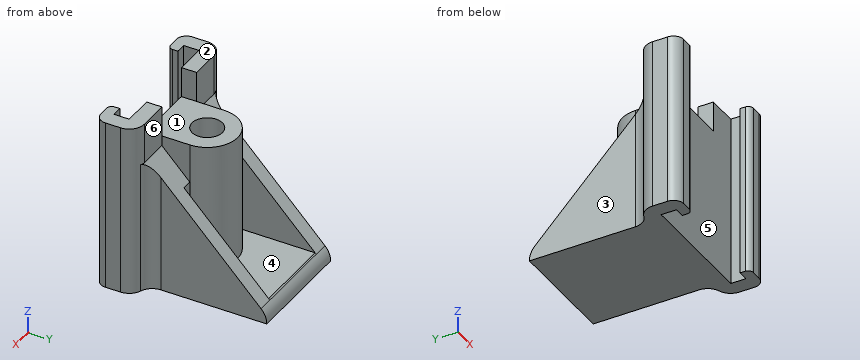
from build123d import *

# Parameters (mm, degrees)
BOSS_EXTRUDE1_DEPTH   = 107.95
BOSS_EXTRUDE1_2_DEPTH = 107.95
SKETCH1_6_W           = 6.35
SKETCH1_6_H           = 17.4625
BOSS_EXTRUDE2_DEPTH   = 82.55
CUT_EXTRUDE2_REACH    = 157.031
BOSS_EXTRUDE4_DEPTH   = 88.9
BOSS_EXTRUDE6_REACH   = 152.176
SKETCH5_R             = 9.525
CUT_EXTRUDE3_DEPTH    = 31.75
FILLET2_R             = 9.525


with BuildPart() as part:
    # Sketch1 → Boss-Extrude1 (new body)
    with BuildSketch(Plane.XY):
        with BuildLine():
            ThreePointArc((34.925, -25.4), (32.67993597, -24.47006403), (31.75, -22.225))
            Line((31.75, -22.225), (31.75, -19.05))
            Line((31.75, -19.05), (38.1, -19.05))
            Line((38.1, -19.05), (38.1, -9.525))
            Line((38.1, -9.525), (19.05, -9.525))
            Line((19.05, -9.525), (19.05, 0))
            Line((19.05, 0), (38.1, 0))
            ThreePointArc((38.1, 0), (44.835192091, -2.789807909), (47.625, -9.525))
            Line((47.625, -9.525), (47.625, -19.05))
            ThreePointArc((47.625, -19.05), (45.765128061, -23.540128061), (41.275, -25.4))
            Line((41.275, -25.4), (34.925, -25.4))
        make_face()
    extrude(amount=BOSS_EXTRUDE1_DEPTH)

    # Sketch1<6> → Boss-Extrude2 (add)
    with BuildSketch(Plane.XY):
        with Locations((22.225, 8.73125)):
            Rectangle(SKETCH1_6_W, SKETCH1_6_H)
        Polygon((25.4, 17.4625), (25.4, 0), (34.925, 0), (34.925, 74.6125), (25.4, 74.6125), align=None)
    boss_extrude2 = extrude(amount=BOSS_EXTRUDE2_DEPTH)

    # Cut-Extrude2: up to this face of the body (flat: up to its plane)
    cut_extrude2_end = Plane(part.part.faces().sort_by_distance((19.05, 3.113443878, 46.562346939))[0])
    # Sketch3 → Cut-Extrude2 (cut, up to the picked face)
    with BuildSketch(Plane(origin=(34.925, 0, 0), x_dir=(0, 0, -1), z_dir=(1, 0, 0)), mode=Mode.PRIVATE) as cut_extrude2_sk1:
        with BuildLine():
            Line((-82.55, 0), (-8.812527697, 71.057408725))
            ThreePointArc((-8.812527697, 71.057408725), (-4.751297675, 73.690240462), (0, 74.6125))
            Line((0, 74.6125), (-82.55, 74.6125))
            Line((-82.55, 74.6125), (-82.55, 0))
        make_face()
    cut_extrude2_tool1 = split(extrude(cut_extrude2_sk1.sketch, amount=-CUT_EXTRUDE2_REACH, mode=Mode.PRIVATE), bisect_by=cut_extrude2_end, keep=Keep.BOTH, mode=Mode.PRIVATE)
    cut_extrude2 = cut_extrude2_tool1.solids().sort_by(Axis((34.925, 49.768554, 56.6833), (-1, 0, 0)))[0]
    add(cut_extrude2, mode=Mode.SUBTRACT)



with BuildPart() as body_2:
    # Sketch1 → Boss-Extrude1 2 (new body)
    with BuildSketch(Plane.XY):
        with BuildLine():
            Line((-38.1, -9.525), (-19.05, -9.525))
            Line((-19.05, -9.525), (-19.05, 0))
            Line((-19.05, 0), (-25.4, 0))
            Line((-25.4, 0), (-34.925, 0))
            Line((-34.925, 0), (-38.1, 0))
            ThreePointArc((-38.1, 0), (-44.835192091, -2.789807909), (-47.625, -9.525))
            Line((-47.625, -9.525), (-47.625, -19.05))
            ThreePointArc((-47.625, -19.05), (-45.765128061, -23.540128061), (-41.275, -25.4))
            Line((-41.275, -25.4), (-34.925, -25.4))
            ThreePointArc((-34.925, -25.4), (-32.67993597, -24.47006403), (-31.75, -22.225))
            Line((-31.75, -22.225), (-31.75, -19.05))
            Line((-31.75, -19.05), (-38.1, -19.05))
            Line((-38.1, -19.05), (-38.1, -9.525))
        make_face()
    extrude(amount=BOSS_EXTRUDE1_2_DEPTH)


with BuildPart() as part_1:
    add(part.part)

    add(body_2.part)  # Boss-Extrude4 merges body 2
    # Sketch1<8> → Boss-Extrude4 (add)
    with BuildSketch(Plane.XY):
        with BuildLine():
            Line((19.05, -9.525), (19.05, 0))
            Line((19.05, 0), (19.05, 17.4625))
            ThreePointArc((19.05, 17.4625), (0, 36.5125), (-19.05, 17.4625))
            Line((-19.05, 17.4625), (-19.05, 0))
            Line((-19.05, 0), (-19.05, -9.525))
            Line((-19.05, -9.525), (19.05, -9.525))
        make_face()
    extrude(amount=BOSS_EXTRUDE4_DEPTH)

    # Mirror1: Boss-Extrude2, Cut-Extrude2 across plane
    add(boss_extrude2.mirror(Plane(origin=(0, 0, 0), x_dir=(0, 0, 1), z_dir=(1, 0, 0))))
    add(cut_extrude2.mirror(Plane(origin=(0, 0, 0), x_dir=(0, 0, 1), z_dir=(1, 0, 0))), mode=Mode.SUBTRACT)

    # Boss-Extrude6: up to this face of the body (flat: up to its plane)
    boss_extrude6_end = Plane(part_1.part.faces().sort_by_distance((25.4, 37.857380573, 21.629312561))[0])
    # Sketch4 → Boss-Extrude6 (add, up to the picked face)
    with BuildSketch(Plane(origin=(-25.4, 0, 0), x_dir=(0, 0, -1), z_dir=(1, 0, 0)), mode=Mode.PRIVATE) as boss_extrude6_sk1:
        with BuildLine():
            Line((0, 17.4625), (0, 74.6125))
            ThreePointArc((0, 74.6125), (-4.751297675, 73.690240462), (-8.812527697, 71.057408725))
            Line((-8.812527697, 71.057408725), (-9.525, 70.312760413))
            Line((-9.525, 70.312760413), (-9.525, 17.4625))
            Line((-9.525, 17.4625), (0, 17.4625))
        make_face()
    boss_extrude6_tool1 = split(extrude(boss_extrude6_sk1.sketch, amount=BOSS_EXTRUDE6_REACH, mode=Mode.PRIVATE), bisect_by=boss_extrude6_end, keep=Keep.BOTH, mode=Mode.PRIVATE)
    add(boss_extrude6_tool1.solids().sort_by(Axis((-25.4, 45.391099, 4.704073), (1, 0, 0)))[0])

    # Sketch5 → Cut-Extrude3 (cut)
    with BuildSketch(Plane.XY.offset(88.9)):
        with Locations((0, 17.4625)):
            Circle(SKETCH5_R)
    extrude(amount=-CUT_EXTRUDE3_DEPTH, mode=Mode.SUBTRACT)

    # Fillet2
    # the kernel refuses this fillet: 9.525 mm, written as the material it adds along each edge
    with BuildSketch(Plane(origin=(-34.925, 0, 0), x_dir=(-0.9963405296085165, -0.08547250469841781, 0), z_dir=(0, 0, 1))) as fillet2_piece_1_section:
        with BuildLine():
            CenterArc((8.769139185, -9.218768342), FILLET2_R, 104.568024357, 70.528779366)
            Line((-0.72100436, -8.404642735), (-1.670018714, -8.323230174))
            Line((-1.670018714, -8.323230174), (-0.949014354, 0.081412561))
            Line((-0.949014354, 0.081412561), (0.081412561, 0.949014354))
            ThreePointArc((0.081412561, 0.949014354), (3.244793742, 0.677639152), (6.133741367, 0.921876834))
            Line((6.133741367, 0.921876834), (6.373322987, 0))
        make_face()
    fillet2_piece_1 = extrude(amount=103.638780605, mode=Mode.PRIVATE)
    fillet2_piece_1 = split(fillet2_piece_1, bisect_by=Plane(origin=(-36.202557182, 22.072398362, 59.645099694), z_dir=(0, -0.7200715531259144, -0.6938998186905898)), keep=Keep.TOP, mode=Mode.PRIVATE)
    add(fillet2_piece_1)
    with BuildSketch(Plane(origin=(34.925, 0, 0), x_dir=(0, 1, 0), z_dir=(0, 0, 1))) as fillet2_piece_2_section:
        with BuildLine():
            CenterArc((8.435512242, -9.525), FILLET2_R, 90, 70.528779366)
            Line((-0.544743879, -6.35), (-1.442769491, -6.0325))
            ThreePointArc((-1.442769491, -6.0325), (-0.9525, -3.175), (-0.9525, 0))
            Line((-0.9525, 0), (0, 0.9525))
            Line((0, 0.9525), (8.435512242, 0.9525))
            Line((8.435512242, 0.9525), (8.435512242, 0))
        make_face()
    fillet2_piece_2 = extrude(amount=103.638780605, mode=Mode.PRIVATE)
    fillet2_piece_2 = split(fillet2_piece_2, bisect_by=Plane(origin=(36.202557182, 22.072398362, 59.645099694), z_dir=(0, -0.7200715531259144, -0.6938998186905898)), keep=Keep.TOP, mode=Mode.PRIVATE)
    add(fillet2_piece_2)


solid = part_1.part
Geometry check sheet. Reference: the model listing, model coordinates, mm. Face numbers are marked on the shaded views. A direction names the side the tool comes from. Round coordinates to 2 decimals unless told otherwise and drop trailing zeros. Write each loop counter-clockwise with the first axis right and the second up, starting at its lowest first coordinate (ties: lowest second). Pieces come first, ordered by that corner, then holes. Notation, with made-up numbers: (9, 32.25) -> (18, 32.25) arc R28 cw to (18, 64.25) -> close; hole circle Ø7 at (22, 73). An arc over 180 degrees is marked (long way). One line per item, written item: value. Start each with the question number.
(1) Scan lines: line 1 (Y direction, x = 0, z = 69) (1 decimal); line 2 (X direction, y = 34, z = 23) (3 decimals); line 3 (X direction, y = -17, z = 43.5) (3 decimals). Record each from-to range of solid material in increasing order. Write a range as [from, to].
(2) Draft check along X on the marked faces 1, 2 and 3. Enter one of: +X half, -X half, draft (parallel to the pull), parting line (faces both ways), or undercut.
(3) Cross-section at B-B, the plane y = 23.5. Record the cut outline in (x, z) (3 decimals).
(4) Go/stop test with flat-tipped pins: pin 1 Ø4 at (x, y) = (-3, -4) entering from -Z; pin 2 Ø3 at (y, z) = (-5.5, 100.5) entering from -X; pin 3 Ø9.5 at (x, z) = (25, 100) entering from +Y; pin 4 Ø15 at (x, y) = (-0.5, 56.5) entering from +Z (3 decimals). Record where each tip stops, or that it passes through.
(5) Access from +Z, -Z, +X, -X, +Y, -Y to the whole of each face (thin tool, end or side, straight path). Record for the marked faces 4, 5 and 6.
Answer:
1. line 1: [-9.5, 7.9], [27, 36.5]
1. line 2: [-34.925, -25.4], [-9.456, 9.456], [25.4, 34.925]
1. line 3: [-47.625, -38.1], [38.1, 47.625]
2. face 1: undercut
2. face 2: draft
2. face 3: -X half
3. outline: (-34.925, 0) -> (34.925, 0) -> (34.925, 58.164) -> (25.4, 58.164) -> (25.4, 9.525) -> (18.068, 9.525) -> (18.068, 88.9) -> (7.367, 88.9) -> (7.367, 57.15) -> (-7.367, 57.15) -> (-7.367, 88.9) -> (-18.068, 88.9) -> (-18.068, 9.525) -> (-25.4, 9.525) -> (-25.4, 58.164) -> (-34.925, 58.164) -> close
4. pin 1: z = 0
4. pin 2: x = -47.28
4. pin 3: y = 0
4. pin 4: z = 9.525
5. face 4: +Z, +Y
5. face 5: +Z, -Z
5. face 6: +Z, +X, +Y
